Source: CAD feature listing. Evaluate the final solid. Frame: model axes, mm. Face numbers are marked on the shaded views. A direction names the side the tool comes from. Coordinates: 2 decimals unless noted, no trailing zeros. Write each loop counter-clockwise with the first axis right and the second up, starting at its lowest first coordinate (ties: lowest second). Pieces come first, ordered by that corner, then holes. Notation, with made-up numbers: M -6,13.5 L 9,13.5 A17 ccw 9,45.5 Z; hole C -34.75,29.5 d4. An arc over 180 degrees is marked long. Answer as CSV lines item,"result". Start each with the question number.
1. Section A-A on y = 35. Return the cut outline in (x, z).
2. Reachability of the marked faces 5, 6, 7, 8 and 9 from +Z, -Z, +X, -X, +Y, -Y: full face, straight path, thin tool, end or side. Return the list, or none.
3. Contact query for flat-ended pins moving along their axis: pin 1 Ø2.5 at (x, z) = (39.5, 5.5) entering from -Y; pin 2 Ø3 at (x, z) = (43, 8.5) entering from +Y. Output: stop coordinate, or through.
4. Section B-B on x = 10.5. Return the cut outline in (y, z).
5. Section C-C on y = -64. Return the cut outline in (x, z).
6. Line query: probe 1 along X at (y, z) = (-67, 4.25); probe 2 along Y at (x, z) = (9, 4); probe 3 along X at (y, z) = (-9.5, 8.25). Output: solid intervals per line, ascending. Write a range as [from, to].
7. Mould query, pull axis X, two halves, no side actions, for the marked faces 1, 2, 3 and 4. Classes: pulls with the +X half, pulls with the -X half, needs draft (parallel to the pull), parting line crosses it, or undercut.
```python
from build123d import *

# Parameters (mm, degrees)
SKETCH2_W           = 110
SKETCH2_H           = 125.38
BOSS_EXTRUDE1_DEPTH = 12.7
FILLET1_R           = 12.8
CUT_EXTRUDE1_DEPTH  = 12.7
BOSS_EXTRUDE2_DEPTH = 12.7


with BuildPart() as part:
    # Sketch2 → Boss-Extrude1 (new body)
    with BuildSketch(Plane.XY):
        with Locations((0, -7.69)):
            Rectangle(SKETCH2_W, SKETCH2_H)
        Polygon((-45, -36.592348927), (-45, 36.592348927), (-36.592348927, 45), (36.592348927, 45), (45, 36.592348927), (45, -36.592348927), (36.592348927, -45), (-36.592348927, -45), align=None, mode=Mode.SUBTRACT)
    extrude(amount=BOSS_EXTRUDE1_DEPTH)

    # Fillet1
    fillet1_edges = [part.edges().sort_by_distance(p)[0] for p in [
        (55, 55, 6.35),
        (-55, 55, 6.35),
    ]]
    fillet(fillet1_edges, radius=FILLET1_R)

    # Sketch5 → Cut-Extrude1 (cut)
    with BuildSketch(Plane(origin=(0, 0, 0), x_dir=(-1, 0, 0), z_dir=(0, 0, -1))):
        Polygon((-38.610878355, -70.38), (-38.610878355, -65.681), (-40.972878355, -65.681), (-40.972878355, -59.839), (-38.610878355, -59.839), (-38.610878355, -55.14), (-32.006878355, -55.14), (-32.006878355, -59.839), (-29.644878355, -59.839), (-29.644878355, -65.681), (-32.006878355, -65.681), (-32.006878355, -70.38), align=None)
        Polygon((32.006878355, -65.681), (32.006878355, -70.38), (38.610878355, -70.38), (38.610878355, -65.681), (40.972878355, -65.681), (40.972878355, -59.839), (38.610878355, -59.839), (38.610878355, -55.14), (32.006878355, -55.14), (32.006878355, -59.839), (29.644878355, -59.839), (29.644878355, -65.681), align=None)
    extrude(amount=-CUT_EXTRUDE1_DEPTH, mode=Mode.SUBTRACT)

    # Sketch6 → Boss-Extrude2 (add)
    with BuildSketch(Plane.XZ.offset(70.38)):
        Polygon((0, 0), (15.875, 0), (15.875, 12.7), (-15.875, 12.7), (-15.875, 0), align=None)
    extrude(amount=BOSS_EXTRUDE2_DEPTH)


solid = part.part
```
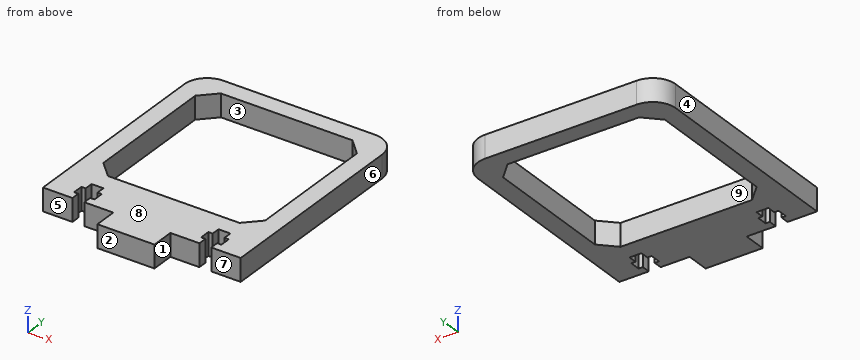
Values:
1,outline,"M -55,0 L -45,0 L -45,12.7 L -55,12.7 Z; M 45,0 L 55,0 L 55,12.7 L 45,12.7 Z"
2,face 5,"+Z, -Z, -X, -Y"
2,face 6,"+Z, -Z, +X, +Y, -Y"
2,face 7,"+Z, -Z, +X, -Y"
2,face 8,"+Z, +X, -X, +Y, -Y"
2,face 9,"+Z, -Z"
3,pin 1,"y = -70.38"
3,pin 2,"y = 55"
4,outline,"M -83.08,0 L -45,0 L -45,12.7 L -83.08,12.7 Z; M 45,0 L 55,0 L 55,12.7 L 45,12.7 Z"
5,outline,"M -55,0 L -40.97,0 L -40.97,12.7 L -55,12.7 Z; M -29.64,0 L 29.64,0 L 29.64,12.7 L -29.64,12.7 Z; M 40.97,0 L 55,0 L 55,12.7 L 40.97,12.7 Z"
6,probe 1,"[-55, -38.61], [-32.01, 32.01], [38.61, 55]"
6,probe 2,"[-83.08, -45], [45, 55]"
6,probe 3,"[-55, -45], [45, 55]"
7,face 1,"pulls with the +X half"
7,face 2,"needs draft"
7,face 3,"undercut"
7,face 4,"pulls with the -X half"
